from build123d import *

# Parameters (mm, degrees)
F0_R     = 5.4
F1_DEPTH = 1.5
F3_DEPTH = 1.5
F5_DEPTH = 1.5
F6_R     = 1
F7_R     = 1
F8_R     = 1


with BuildPart() as f1:
    # F0 (on Front) → F1 (new body, symmetric)
    with BuildSketch(Plane.XZ):
        Circle(F0_R)
        with BuildLine():
            ThreePointArc((1.525, 2.1057955741), (2.3157072354, 1.1821590418), (2.6, 0))
            ThreePointArc((2.6, 0), (2.3157072354, -1.1821590418), (1.525, -2.1057955741))
            ThreePointArc((1.525, -2.1057955741), (0, -2.6), (-1.525, -2.1057955741))
            ThreePointArc((-1.525, -2.1057955741), (-2.6, 0), (-1.525, 2.1057955741))
            ThreePointArc((-1.525, 2.1057955741), (0, 2.6), (1.525, 2.1057955741))
        make_face(mode=Mode.SUBTRACT)
        with BuildLine():
            Line((-1.525, -2.1057955741), (-1.525, 2.1057955741))
            ThreePointArc((-1.525, 2.1057955741), (-2.6, 0), (-1.525, -2.1057955741))
        make_face()
        with BuildLine():
            ThreePointArc((1.525, -2.1057955741), (2.3157072354, -1.1821590418), (2.6, 0))
            ThreePointArc((2.6, 0), (2.3157072354, 1.1821590418), (1.525, 2.1057955741))
            Line((1.525, 2.1057955741), (1.525, -2.1057955741))
        make_face()
    extrude(amount=F1_DEPTH, both=True)

    # F2 (on Front) → F3 (join, through all)
    with BuildSketch(Plane.XZ):
        Polygon((-0.9291996635, 4.3362903498), (0, 4.3362903498), (0, 35), (-2, 35), align=None)
        Polygon((0, 35), (0, 4.3362903498), (0.9291996635, 4.3362903498), (2, 35), align=None)
    extrude(amount=-F3_DEPTH)

    # F4 (on Front) → F5 (join, through all)
    with BuildSketch(Plane.XZ):
        Polygon((0, 35), (0, 47.5), (-7.5, 35), align=None)
        Polygon((7.5, 35), (0, 47.5), (0, 35), align=None)
    extrude(amount=-F5_DEPTH)

    # F6
    f6_edges = [f1.edges().sort_by_distance(p)[0] for p in [
        (7.5, 0.75, 35),
    ]]
    fillet(f6_edges, radius=F6_R)

    # F7
    f7_edges = [f1.edges().sort_by_distance(p)[0] for p in [
        (0, 0.75, 47.5),
    ]]
    fillet(f7_edges, radius=F7_R)

    # F8
    f8_edges = [f1.edges().sort_by_distance(p)[0] for p in [
        (-7.5, 0.75, 35),
    ]]
    fillet(f8_edges, radius=F8_R)


solid = f1.part
CAD build for the part. Positions are in the model's coordinates, mm. A direction names the side the tool comes from. Give positions to 0.01 mm unless a question says otherwise; leave off trailing zeros. Write each loop counter-clockwise with the first axis right and the second up, starting at its lowest first coordinate (ties: lowest second). Pieces come first, ordered by that corner, then holes. Notation, with made-up numbers: (26, -2) -> (79, -2) arc R24 ccw to (79, 27) -> close; hole circle Ø1 at (-3, 25.25). An arc over 180 degrees is marked (long way). Return JSON: item names as keys, results as strings.
Item 1: Band-saw the part on A-A (z = 0). List the corners of the cut face in (x, y) (3 decimals), then the cut area to 4 significant figures.
Answer below:
{"outline": "(-5.4, -1.5) -> (-1.525, -1.5) -> (-1.525, 1.5) -> (-5.4, 1.5) -> close; (1.525, -1.5) -> (5.4, -1.5) -> (5.4, 1.5) -> (1.525, 1.5) -> close", "area": "23.25 mm2"}
Item 2: Drill centre lines: probe 1 along Y at (x, z) = (-1.25, 23); probe 2 along X at (y, z) = (-1, -1) (3 decimals); probe 3 along Z at (x, y) = (2.25, 0.85). Where is each one in solid material? Low to high.
Answer below:
{"probe 1": "y = 0 to 1.5", "probe 2": "x = -5.307 to -1.525, 1.525 to 5.307", "probe 3": "z = -4.91 to 4.91, 35 to 43.75"}
Item 3: Tool access for faces 1 (the flat face through (0, 0, 31)), 2 (the flat face through (-4, 1, 35)), 3 (the flat face through (3.76, 0.74, 41.23)), 4 (the cylindrical face through (0, 0, 2.6)), 5 (the flat face through (4, 1, 35)): list every direction of +Z, -Z, +X, -X, +Y, -Y with a clear straight run to the whole face (end or side of a thin tool).
Answer below:
{"face 1": "+Z, +X, -X, -Y", "face 2": "-X, +Y, -Y", "face 3": "+Z, +X, +Y, -Y", "face 4": "+Y, -Y", "face 5": "+X, +Y, -Y"}
Item 4: Drop flat-ended pins along their axis: pin 1 (1.5 mm diameter, centred on y = 0, z = -1, fed in from +X); pin 2 (6 mm diameter, centred on x = 0, z = 8.5, fed in from -Y); pin 3 (1.2 mm diameter, centred on x = -3.5, y = 1, fed in from -Z). Give the stop position or say it passes through.
Answer below:
{"pin 1": "stops at x = 5.39", "pin 2": "stops at y = 0", "pin 3": "stops at z = -4.56"}
Item 5: Band-saw the part on D-D (z = 37). List the corners of the cut face in (x, y).
Answer below:
{"outline": "(-6.3, 0) -> (6.3, 0) -> (6.3, 1.5) -> (-6.3, 1.5) -> close"}
Item 6: Band-saw the part on C-C (y = -1.05). List the corners of the cut face in (x, z) (3 decimals).
Answer below:
{"outline": "circle Ø10.8 at (0, 0); hole (-1.525, -2.106) arc R2.6 ccw to (1.525, -2.106) -> (1.525, 2.106) arc R2.6 ccw to (-1.525, 2.106) -> close"}
Item 7: Band-saw the part on B-B (x = 0). List the corners of the cut face in (y, z).
Answer below:
{"outline": "(-1.5, -5.4) -> (1.5, -5.4) -> (1.5, -2.6) -> (-1.5, -2.6) -> close; (-1.5, 2.6) -> (1.5, 2.6) -> (1.5, 46.56) -> (0, 46.56) -> (0, 5.4) -> (-1.5, 5.4) -> close"}
